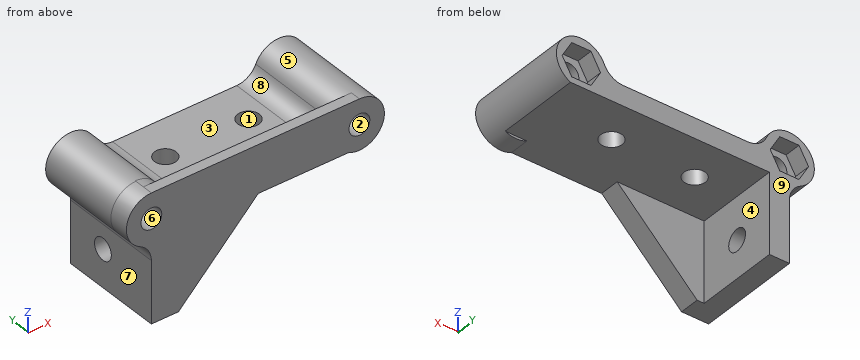
from build123d import *
from build123d.topology import SkipClean

# Parameters (mm, degrees)
BOSS_EXTRUDE1_DEPTH = 4.8
BOSS_EXTRUDE2_DEPTH = 20.2
BOSS_EXTRUDE3_DEPTH = 0.2
CHAMFER1_SIZE       = 2.5
SKETCH4_R           = 2.5
CUT_EXTRUDE1_DEPTH  = 67.076924868
CUT_EXTRUDE2_DEPTH  = 4
SKETCH6_R           = 2.6
CUT_EXTRUDE3_DEPTH  = 65.262275092
SKETCH7_R           = 2.6
CUT_EXTRUDE4_DEPTH  = 63.061260058


with BuildPart() as part:
    # Sketch1 → Boss-Extrude1 (new body)
    with BuildSketch(Plane(origin=(0, 0, 0), x_dir=(1, 0, 0), z_dir=(0, 1, 0))):
        with BuildLine():
            Line((0, -6), (50, -6))
            ThreePointArc((50, -6), (55.848076607, 1.341640786), (47.384660634, 5.4))
            Line((47.384660634, 5.4), (25.7, 5.4))
            Line((25.7, 5.4), (6.5, 24.6))
            Line((6.5, 24.6), (0, 24.6))
            Line((0, 24.6), (0, 9.797958971))
            ThreePointArc((0, 9.797958971), (-0.735985673, 7.186794132), (-2.727272727, 5.344341257))
            ThreePointArc((-2.727272727, 5.344341257), (-5.833782973, -1.402489297), (0, -6))
        make_face()
    extrude(amount=BOSS_EXTRUDE1_DEPTH)

    # Sketch2 → Boss-Extrude2 (add)
    with SkipClean():  # the faces are left unmerged after this step: merging them gives an invalid solid
        with BuildSketch(Plane(origin=(0, 4.8, 0), x_dir=(1, 0, 0), z_dir=(0, 1, 0))):
            with BuildLine():
                Line((0, 24.6), (4.8, 24.6))
                Line((4.8, 24.6), (4.8, 5.4))
                Line((4.8, 5.4), (52.615339366, 5.4))
                ThreePointArc((52.615339366, 5.4), (54.158005006, -4.325620692), (44.500909166, -2.4))
                ThreePointArc((44.500909166, -2.4), (42.656946259, -0.216699867), (39.918333471, 0.6))
                Line((39.918333471, 0.6), (10.081666529, 0.6))
                ThreePointArc((10.081666529, 0.6), (7.343053741, -0.216699867), (5.499090834, -2.4))
                ThreePointArc((5.499090834, -2.4), (-4.112717992, -4.368701262), (-2.727272727, 5.344341257))
                ThreePointArc((-2.727272727, 5.344341257), (-0.735985673, 7.186794132), (0, 9.797958971))
                Line((0, 9.797958971), (0, 24.6))
            make_face()
        extrude(amount=BOSS_EXTRUDE2_DEPTH)

    # Sketch3 → Boss-Extrude3 (add)
    with SkipClean():  # the faces are left unmerged after this step: merging them gives an invalid solid
        with BuildSketch(Plane(origin=(0, 4.8, 0), x_dir=(1, 0, 0), z_dir=(0, 1, 0))):
            with BuildLine():
                Line((39.918333471, 0.6), (10.081666529, 0.6))
                ThreePointArc((10.081666529, 0.6), (7.343053741, -0.216699867), (5.499090834, -2.4))
                ThreePointArc((5.499090834, -2.4), (3.286335345, -5.019960159), (0, -6))
                Line((0, -6), (50, -6))
                ThreePointArc((50, -6), (46.713664655, -5.019960159), (44.500909166, -2.4))
                ThreePointArc((44.500909166, -2.4), (42.656946259, -0.216699867), (39.918333471, 0.6))
            make_face()
        extrude(amount=BOSS_EXTRUDE3_DEPTH)

    # Chamfer1
    # the kernel refuses this chamfer: 2.5 mm, written as the material it takes off along each edge
    with BuildSketch(Plane(origin=(-6.42920747, 5, 6), x_dir=(0, -0.9996219169112968, 0.027495876610586317), z_dir=(1, 0, 0))) as chamfer1_piece_1_section:
        Polygon((CHAMFER1_SIZE * 0.999621916911, CHAMFER1_SIZE * 0.0274958766106), (-CHAMFER1_SIZE * 0.0274958766106, CHAMFER1_SIZE * 0.999621916911), (0, 0), align=None)
    chamfer1_piece_1 = extrude(amount=62.85841494, mode=Mode.PRIVATE)
    chamfer1_piece_1 = chamfer1_piece_1 - Plane(origin=(0, 4.144274293, 0), x_dir=(0.9165151389911681, 0, 0.3999999999999999), z_dir=(0, -1, 0)) * Cylinder(6, 136, mode=Mode.PRIVATE)
    chamfer1_piece_1 = chamfer1_piece_1 - Plane(origin=(50, 4.144274293, 0), x_dir=(0.43588989435406716, 0, -0.9000000000000001), z_dir=(0, -1, 0)) * Cylinder(6, 136, mode=Mode.PRIVATE)
    add(chamfer1_piece_1, mode=Mode.SUBTRACT)

    # Sketch4 → Cut-Extrude1 (cut, through all)
    with BuildSketch(Plane.XZ):
        with Locations(Location((0, 0, 0), (0, 0, 270))):
            Circle(SKETCH4_R)
        with Locations(Location((50, 0, 0), (0, 0, 270))):
            Circle(SKETCH4_R)
    extrude(amount=-CUT_EXTRUDE1_DEPTH, mode=Mode.SUBTRACT)

    # Sketch5 → Cut-Extrude2 (cut)
    with BuildSketch(Plane(origin=(0, 25, 0), x_dir=(1, 0, 0), z_dir=(0, 1, 0))):
        Polygon((4.618802154, 0), (2.309401077, 4), (-2.309401077, 4), (-4.618802154, 0), (-2.309401077, -4), (2.309401077, -4), align=None)
        Polygon((47.690598923, 4), (45.381197846, 0), (47.690598923, -4), (52.309401077, -4), (54.618802154, 0), (52.309401077, 4), align=None)
    extrude(amount=-CUT_EXTRUDE2_DEPTH, mode=Mode.SUBTRACT)

    # Sketch6 → Cut-Extrude3 (cut, through all)
    with BuildSketch(Plane(origin=(0, 0, -5.4), x_dir=(-1, 0, 0), z_dir=(0, 0, -1))):
        with Locations((-35, 15)):
            Circle(SKETCH6_R)
        with Locations((-15, 15)):
            Circle(SKETCH6_R)
    extrude(amount=-CUT_EXTRUDE3_DEPTH, mode=Mode.SUBTRACT)

    # Sketch7 → Cut-Extrude4 (cut, through all)
    with BuildSketch(Plane(origin=(4.8, 0, 0), x_dir=(0, 0, -1), z_dir=(1, 0, 0))):
        with Locations((15.6, 15)):
            Circle(SKETCH7_R)
    extrude(amount=-CUT_EXTRUDE4_DEPTH, mode=Mode.SUBTRACT)


solid = part.part
Work out the finished part from the listing and answer in its coordinate system (mm). Face numbers are marked on the shaded views. A direction names the side the tool comes from. Round coordinates to 2 decimals unless told otherwise and drop trailing zeros. Write each loop counter-clockwise with the first axis right and the second up, starting at its lowest first coordinate (ties: lowest second). Pieces come first, ordered by that corner, then holes. Notation, with made-up numbers: (15.25, 20.5) -> (28.25, 20.5) arc R23 ccw to (28.25, 53.5) -> close; hole circle Ø7 at (-3.75, 11). An arc over 180 degrees is marked (long way). Answer as CSV lines item,"result". Start each with the question number.
(1) Each of these flat-tipped pins is pushed along its axis until it touches: pin 1 (1.5 mm diameter, centred on x = 7, z = -6.5, fed in from -Y); pin 2 (1.2 mm diameter, centred on x = 24.5, z = 1, fed in from +Y); pin 3 (3 mm diameter, centred on y = 5.5, z = -13, fed in from +X); pin 4 (4.5 mm diameter, centred on y = 17.5, z = -15, fed in from -X). Where does it stop, or does it pass through?
(2) The part is cut by section C-C, the plane x = 15. Give the vertices of the cut face in (y, z), then the cut area to 3 significant figures.
(3) The mould has two halves that part along X. Classify the marked faces 6, 7, 8 and 9: +X half, -X half, draft (parallel to the pull), parting line (faces both ways), or undercut.
(4) Find the intervals of material crossed by probe 1 along Y at (x, z) = (35, -4.2); probe 2 along X at (y, z) = (14.5, 0); probe 3 along X at (y, z) = (13.25, -2), in increasing order.
(5) The part is cut by section A-A, the plane y = 15. Give the vertices of the cut face in (x, z).
(6) A tool of negligible diameter and unlimited length cuts with its end or side. For the marked faces 1, 2, 3, 4 and 5, from which of +Z, -Z, +X, -X, +Y, -Y can it reach the whole face along a straight path? Write none if from no direction.
(7) The part is cut by section B-B, the plane z = -15.6. Give the vertices of the cut face in (x, y), then the cut area to 3 significant figures.
(8) The part is cut by section D-D, the plane y = 19.75. Give the vertices of the cut face in (x, z).
Output values:
1,pin 1,"stops at y = 0"
1,pin 2,"stops at y = 5"
1,pin 3,"stops at x = 19.43"
1,pin 4,"stops at x = 0"
2,outline,"(0, -16.1) -> (4.8, -16.1) -> (4.8, -5.4) -> (12.4, -5.4) -> (12.4, -0.6) -> (5, -0.6) -> (5, 3.5) -> (2.5, 6) -> (0, 6) -> close; (17.6, -5.4) -> (25, -5.4) -> (25, -0.6) -> (17.6, -0.6) -> close"
2,area,"176 mm²"
3,face 6,"undercut"
3,face 7,"-X half"
3,face 8,"undercut"
3,face 9,"draft"
4,probe 1,"y = 0 to 12.4, 17.6 to 25"
4,probe 2,"x = -6 to -2.5, 2.5 to 7.71, 42.29 to 47.5, 52.5 to 56"
4,probe 3,"x = -5.66 to -1.5, 1.5 to 13.08, 16.92 to 33.08, 36.92 to 48.5, 51.5 to 55.66"
5,outline,"(-2.73, -5.34) arc R5 cw to (0, -9.8) -> (0, -13) -> (4.8, -13) -> (4.8, -5.4) -> (12.4, -5.4) -> (12.4, -0.6) -> (10.08, -0.6) arc R5 cw to (5.5, 2.4) arc R6 ccw (long way) to start; (0, -24.6) -> (4.8, -24.6) -> (4.8, -18.2) -> (0, -18.2) -> close; (17.6, -5.4) -> (32.4, -5.4) -> (32.4, -0.6) -> (17.6, -0.6) -> close; (37.6, -5.4) -> (52.62, -5.4) arc R6 ccw (long way) to (44.5, 2.4) arc R5 cw to (39.92, -0.6) -> (37.6, -0.6) -> close; hole circle Ø5 at (0, 0); hole circle Ø5 at (50, 0)"
6,face 1,"+Z, -Z"
6,face 2,"+Y, -Y"
6,face 3,"+Z, +Y"
6,face 4,"-Z, +X, +Y"
6,face 5,"+Y"
7,outline,"(0, 0) -> (15.5, 0) -> (15.5, 4.8) -> (4.8, 4.8) -> (4.8, 12.4) -> (0, 12.4) -> close; (0, 17.6) -> (4.8, 17.6) -> (4.8, 25) -> (0, 25) -> close"
7,area,"146 mm²"
8,outline,"(-2.73, -5.34) arc R5 cw to (0, -9.8) -> (0, -24.6) -> (4.8, -24.6) -> (4.8, -5.4) -> (52.62, -5.4) arc R6 ccw (long way) to (44.5, 2.4) arc R5 cw to (39.92, -0.6) -> (10.08, -0.6) arc R5 cw to (5.5, 2.4) arc R6 ccw (long way) to start; hole circle Ø5 at (0, 0); hole circle Ø5 at (50, 0)"
